Can you work these out from the model? Positions are in its coordinate system, mm. A direction names the side the tool comes from. Round coordinates to 2 decimals unless told otherwise and drop trailing zeros. Write each loop counter-clockwise with the first axis right and the second up, starting at its lowest first coordinate (ties: lowest second). Pieces come first, ordered by that corner, then holes. Notation, with made-up numbers: (-37.75, 16) -> (-20.75, 16) arc R20 cw to (-20.75, 37) -> close; hole circle Ø11 at (12, 34.25). An arc over 180 degrees is marked (long way). Use CSV: the item, a comma, the result in double quotes.
```python
from build123d import *

# Parameters (mm, degrees)
SKETCH_1_W          = 25
SKETCH_1_H          = 140
EXTRUDE_1_DEPTH     = 4
FILLET_1_R          = 2
SKETCH_4_R          = 1.75
CUT_EXTRUDE_1_DEPTH = 10
SKETCH_6_W          = 3
SKETCH_6_H          = 140
EXTRUDE_3_DEPTH     = 1.5
SKETCH_7_W          = 20.611875048
SKETCH_7_H          = 50
CUT_EXTRUDE_2_DEPTH = 10
SKETCH_8_W          = 3.5
SKETCH_8_H          = 50
CUT_EXTRUDE_3_DEPTH = 45


with BuildPart() as part:
    # 草图1 → 凸台-拉伸1 (new body)
    with BuildSketch(Plane(origin=(0, 0, 0), x_dir=(1, 0, 0), z_dir=(0, 1, 0))):
        Rectangle(SKETCH_1_W, SKETCH_1_H)
    extrude(amount=EXTRUDE_1_DEPTH)

    # 圆角1
    fillet_1_edges = [part.edges().sort_by_distance(p)[0] for p in [
        (12.5, 2, 70),
        (-12.5, 2, 70),
        (-12.5, 2, -70),
        (12.5, 2, -70),
    ]]
    fillet(fillet_1_edges, radius=FILLET_1_R)

    # 草图4 → 切除-拉伸1 (cut)
    with BuildSketch(Plane(origin=(0, 4, 0), x_dir=(1, 0, 0), z_dir=(0, 1, 0))):
        with Locations(Location((0, 60, 0), (0, 0, 270))):
            Circle(SKETCH_4_R)
        with Locations(Location((0, -60, 0), (0, 0, 90))):
            Circle(SKETCH_4_R)
    extrude(amount=-CUT_EXTRUDE_1_DEPTH, mode=Mode.SUBTRACT)

    # 草图6 → 凸台-拉伸3 (add)
    with BuildSketch(Plane(origin=(0, 4, 0), x_dir=(1, 0, 0), z_dir=(0, 1, 0))):
        with Locations((6, 0)):
            Rectangle(SKETCH_6_W, SKETCH_6_H)
    extrude(amount=EXTRUDE_3_DEPTH)

    # 草图7 → 切除-拉伸2 (cut)
    with BuildSketch(Plane(origin=(0, 4, 0), x_dir=(1, 0, 0), z_dir=(0, 1, 0))):
        with Locations((-17.805937524, 45)):
            Rectangle(SKETCH_7_W, SKETCH_7_H)
    extrude(amount=-CUT_EXTRUDE_2_DEPTH, mode=Mode.SUBTRACT)

    # 草图8 → 切除-拉伸3 (cut)
    with BuildSketch(Plane(origin=(0, 4, 0), x_dir=(1, 0, 0), z_dir=(0, 1, 0))):
        with Locations((10.75, -45)):
            Rectangle(SKETCH_8_W, SKETCH_8_H)
    extrude(amount=-CUT_EXTRUDE_3_DEPTH, mode=Mode.SUBTRACT)


solid = part.part
```
Q1. Suppose I cut it at A-A (x = 0). Write out the boundary of the cut face in (y, z).
Resolved:
outline,"(0, -70) -> (4, -70) -> (4, -61.75) -> (0, -61.75) -> close; (0, -58.25) -> (4, -58.25) -> (4, 58.25) -> (0, 58.25) -> close; (0, 61.75) -> (4, 61.75) -> (4, 70) -> (0, 70) -> close"
Q2. On a 3-axis mill with a long thin cutter (end or side, diameter ignored), from which of +Z, -Z, +X, -X, +Y, -Y can I reach the whole of each face in a straight line? I mean faces 1 (the face through (10, 4, -17)), 2 (the face through (9, 2, 45)), 3 (the face through (-7.5, 2, -45)). Say none if no direction works.
Resolved:
face 1,"+Z, -Z, +X, +Y"
face 2,"+Z, +X, +Y, -Y"
face 3,"-Z, -X, +Y, -Y"
Q3. Suppose I cut it at D-D (z = 40.5). Write out the boundary of the cut face in (x, y), and give its area (3 significant figures).
Resolved:
outline,"(-12.5, 0) -> (9, 0) -> (9, 4) -> (7.5, 4) -> (7.5, 5.5) -> (4.5, 5.5) -> (4.5, 4) -> (-12.5, 4) -> close"
area,"90.5 mm^2"
Q4. Suppose I cut it at B-B (z = -60). Write out the boundary of the cut face in (x, y), and give its area (3 significant figures).
Resolved:
outline,"(-7.5, 0) -> (-1.75, 0) -> (-1.75, 4) -> (-7.5, 4) -> close; (1.75, 0) -> (12.5, 0) -> (12.5, 4) -> (7.5, 4) -> (7.5, 5.5) -> (4.5, 5.5) -> (4.5, 4) -> (1.75, 4) -> close"
area,"70.5 mm^2"
Q5. If we mould it in two halves opening along Z, with no side actions, what happens to faces 4 (the face through (-12.5, 2, 25)), 5 (the face through (-1, 2, 70)), 6 (the face through (0.67, 2.028, 58.383))? For each: released by +Z, released by -Z, zero draft, split by the parting line, or undercut.
Resolved:
face 4,"zero draft"
face 5,"released by +Z"
face 6,"undercut"
Q6. Suppose I cut it at C-C (y = 1.55). Write out the boundary of the cut face in (x, z), and give its area (3 significant figures).
Resolved:
outline,"(-12.5, -20) -> (-7.5, -20) -> (-7.5, -70) -> (10.5, -70) arc R2 ccw to (12.5, -68) -> (12.5, 20) -> (9, 20) -> (9, 70) -> (-10.5, 70) arc R2 ccw to (-12.5, 68) -> close; hole circle Ø3.5 at (0, -60); hole circle Ø3.5 at (0, 60)"
area,"3,050 mm^2"
Q7. Please list where these lines run through material, in increasing order: probe 1 along Z at (x, y) = (0.25, 1.9); probe 2 along X at (y, z) = (1.5, 60); probe 3 along X at (y, z) = (2.45, -60).
Resolved:
probe 1,"z = -70 to -61.73, -58.27 to 58.27, 61.73 to 70"
probe 2,"x = -12.5 to -1.75, 1.75 to 9"
probe 3,"x = -7.5 to -1.75, 1.75 to 12.5"
Q8. Will these pins go through, and if not, where does the flat tip stop? P1, Ø3, axis at x = -11, y = 2.5, coming from the -Z side; P2, Ø10, axis at x = -7, z = -33, coming from the -Y side; P3, Ø2, axis at y = 2, z = -53, coming from the -X side; P4, Ø0.8, axis at y = 4.5, z = -0.5, coming from the -X side.
Resolved:
P1,"stops at z = -20"
P2,"stops at y = 0"
P3,"stops at x = -7.5"
P4,"stops at x = 4.5"
